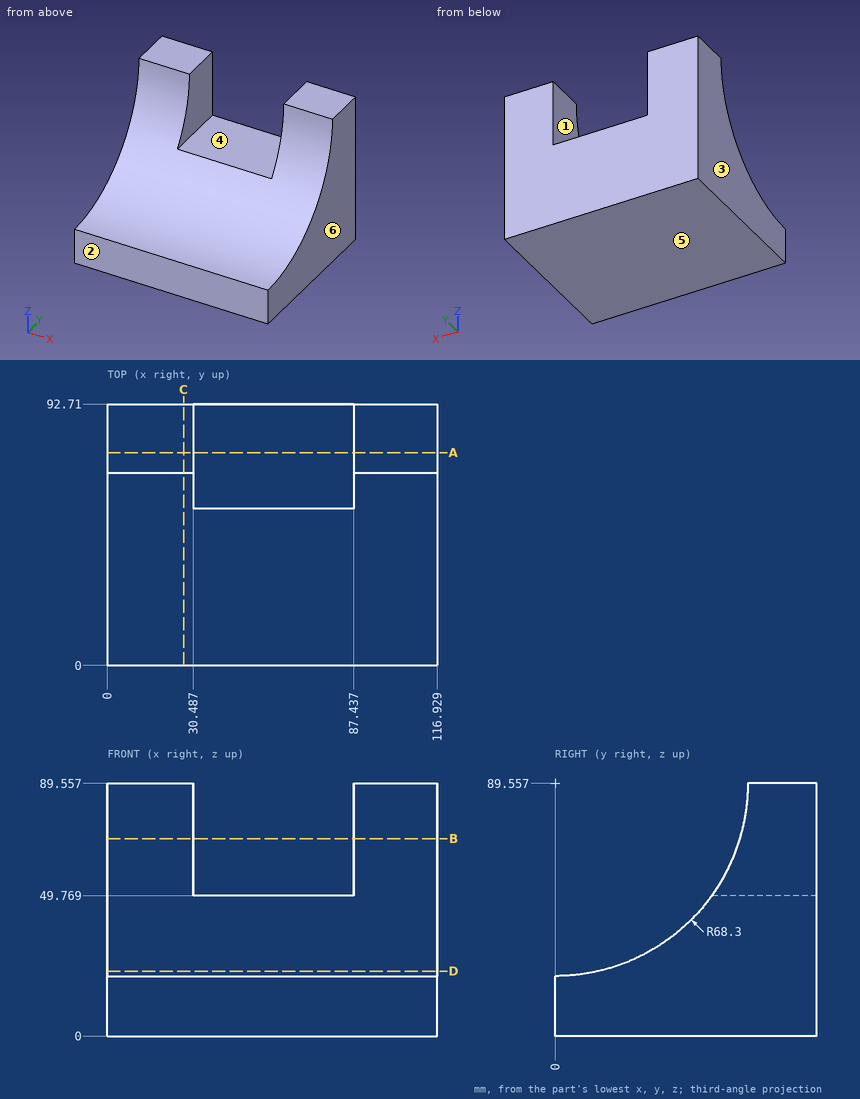
Geometry check sheet. Reference: drawing and pictorial views, mm from the part's lowest x, y, z. A direction names the side the tool comes from. Coordinates: 2 decimals unless noted, no trailing zeros. Write each loop counter-clockwise with the first axis right and the second up, starting at its lowest first coordinate (ties: lowest second). Pieces come first, ordered by that corner, then holes. Notation, with made-up numbers: M 57,66.5 L 102,66.5 A11 cw 102,85.5 Z; hole C 18.25,73.5 d2. An arc over 180 degrees is marked long. Use one line per item in the form item = value.
Item 1: Sectioned sample at A-A, the plane y = 75.5. Record the cut outline in (x, z), and give its area (3 significant figures).
Answer below:
outline = M 0,0 L 116.93,0 L 116.93,89.56 L 87.44,89.56 L 87.44,49.77 L 30.49,49.77 L 30.49,89.56 L 0,89.56 Z
area = 8,210 mm^2
Item 2: Set-up check for the marked faces 1 and 2: record each of +Z, -Z, +X, -X, +Y, -Y from which the full face is reachable in a straight line by a thin tool's end or side.
Answer below:
face_1 = +Z, +Y, -Y
face_2 = +Z, -Z, +X, -X, -Y
Item 3: Release check for a two-part mould opening along X. For the marked faces 3, 4, 5 and 6 record: pulls with the +X half, pulls with the -X half, needs draft (parallel to the pull), parting line crosses it, or undercut.
Answer below:
face_3 = pulls with the -X half
face_4 = undercut
face_5 = needs draft
face_6 = pulls with the +X half
Item 4: Sectioned sample at B-B, the plane z = 70. Record the cut outline in (x, y).
Answer below:
outline = M 0,65.44 L 30.49,65.44 L 30.49,92.71 L 0,92.71 Z; M 87.44,65.44 L 116.93,65.44 L 116.93,92.71 L 87.44,92.71 Z
Item 5: Sectioned sample at C-C, the plane x = 27. Record the cut outline in (y, z).
Answer below:
outline = M 0,0 L 92.71,0 L 92.71,89.56 L 68.3,89.56 A68.3 cw 0,21.26 Z
Item 6: Gauge pin test, flat ends, axial feed: pin 1 Ø12 at (x, y) = (62.5, 68.5) entering from -Z; pin 2 Ø1 at (x, y) = (63, 56.5) entering from +Z; pin 3 Ø2 at (x, y) = (87, 22.5) entering from +Z. Record the tip position at first contact, or that the pin passes through.
Answer below:
pin_1 = 0
pin_2 = 49.77
pin_3 = 25.43
Item 7: Sectioned sample at D-D, the plane z = 23. Record the cut outline in (x, y).
Answer below:
outline = M 0,15.33 L 116.93,15.33 L 116.93,92.71 L 0,92.71 Z
Item 8: Material ranges on L1, parallel to X at y = 84, z = 73.5; L2, parallel to Z at x = 83.5, y = 72; L3, parallel to Z at x = 7.5, y = 23.5, recorded low to high. Write a range as from..to.
Answer below:
L1 = 0..30.49, 87.44..116.93
L2 = 0..49.77
L3 = 0..25.43
